Source: CAD feature listing. Evaluate the final solid. Frame: model axes, mm. A direction names the side the tool comes from. Round coordinates to 2 decimals unless told otherwise and drop trailing zeros. Write each loop counter-clockwise with the first axis right and the second up, starting at its lowest first coordinate (ties: lowest second). Pieces come first, ordered by that corner, then holes. Notation, with made-up numbers: M 8,55 L 33,55 A10 ccw 33,64 Z; hole C 48,54.25 d3. An arc over 180 degrees is marked long. Put each result on its own line as item: value. Start each with the question number.
```python
from build123d import *

# Parameters (mm, degrees)
SKETCH1_W           = 132
SKETCH1_H           = 87
SKETCH1_W_2         = 100
SKETCH1_H_2         = 55
BOSS_EXTRUDE1_DEPTH = 256
CUT_EXTRUDE1_REACH  = 89
SKETCH4_W           = 80
SKETCH4_H           = 70
CUT_EXTRUDE2_REACH  = 89
SKETCH5_W           = 70
SKETCH5_H           = 70
SKETCH6_W           = 100
SKETCH6_H           = 55
BOSS_EXTRUDE2_DEPTH = 16
SKETCH7_W           = 106
SKETCH7_H           = 17.5
CUT_EXTRUDE3_DEPTH  = 133
SKETCH9_W           = 106
SKETCH9_H           = 7.5
BOSS_EXTRUDE4_DEPTH = 16
CUT_EXTRUDE4_REACH  = 134
SKETCH10_R          = 12.5


with BuildPart() as part:
    # Sketch1 → Boss-Extrude1 (new body)
    with BuildSketch(Plane.XY):
        with Locations((-66, 43.5)):
            Rectangle(SKETCH1_W, SKETCH1_H)
        with Locations((-66, 43.5)):
            Rectangle(SKETCH1_W_2, SKETCH1_H_2, mode=Mode.SUBTRACT)
    extrude(amount=BOSS_EXTRUDE1_DEPTH)

    # Sketch4 → Cut-Extrude1 (cut, up to next)
    with BuildSketch(Plane(origin=(0, 87, 0), x_dir=(1, 0, 0), z_dir=(0, 1, 0)), mode=Mode.PRIVATE) as cut_extrude1_sk1:
        with Locations((-66, -201)):
            Rectangle(SKETCH4_W, SKETCH4_H)
    cut_extrude1_tool1 = extrude(cut_extrude1_sk1.sketch, amount=-CUT_EXTRUDE1_REACH, mode=Mode.PRIVATE) & part.part
    add(cut_extrude1_tool1.solids().sort_by_distance((-66, 87, 201))[0], mode=Mode.SUBTRACT)

    # Sketch5 → Cut-Extrude2 (cut, up to next)
    with BuildSketch(Plane(origin=(0, 87, 0), x_dir=(1, 0, 0), z_dir=(0, 1, 0)), mode=Mode.PRIVATE) as cut_extrude2_sk1:
        with Locations((-66, -51)):
            Rectangle(SKETCH5_W, SKETCH5_H)
    cut_extrude2_tool1 = extrude(cut_extrude2_sk1.sketch, amount=-CUT_EXTRUDE2_REACH, mode=Mode.PRIVATE) & part.part
    add(cut_extrude2_tool1.solids().sort_by_distance((-66, 87, 51))[0], mode=Mode.SUBTRACT)

    # Sketch6 → Boss-Extrude2 (add)
    with BuildSketch(Plane(origin=(0, 0, 0), x_dir=(-1, 0, 0), z_dir=(0, 0, -1))):
        with Locations((66, 43.5)):
            Rectangle(SKETCH6_W, SKETCH6_H)
    extrude(amount=-BOSS_EXTRUDE2_DEPTH)

    # Sketch7 → Cut-Extrude3 (cut, through all)
    with BuildSketch(Plane(origin=(0, 0, 0), x_dir=(0, 0, -1), z_dir=(1, 0, 0))):
        with Locations((-53, 8.75)):
            Rectangle(SKETCH7_W, SKETCH7_H)
    extrude(amount=-CUT_EXTRUDE3_DEPTH, mode=Mode.SUBTRACT)

    # Sketch9 → Boss-Extrude4 (add)
    with BuildSketch(Plane.ZY.offset(132)):
        with Locations((53, 13.75)):
            Rectangle(SKETCH9_W, SKETCH9_H)
    extrude(amount=-BOSS_EXTRUDE4_DEPTH)

    # Sketch10 → Cut-Extrude4 (cut, up to next)
    with BuildSketch(Plane.ZY.offset(132), mode=Mode.PRIVATE) as cut_extrude4_sk1:
        with Locations((201, 57.5)):
            Circle(SKETCH10_R)
    cut_extrude4_tool1 = extrude(cut_extrude4_sk1.sketch, amount=-CUT_EXTRUDE4_REACH, mode=Mode.PRIVATE) & part.part
    add(cut_extrude4_tool1.solids().sort_by_distance((-132, 57.5, 201))[0], mode=Mode.SUBTRACT)


solid = part.part
```
(1) Section query B-B (x = -18.5). Return loops of the section in (y, z), and give its area (3 significant figures).
(2) Pull-direction query (X, two-part tool) for faces 1 (the flat face through (-67, 87, 126)), 2 (the flat face through (-67, 53, 16)), 3 (the flat face through (-132, 44, 126)); classes: +X half, -X half, draft (parallel to the pull), parting line (faces both ways), or undercut.
(3) Ray query, line 1 along X through (y, z) = (58, 136); line 2 along Y through (x, z) = (-127, 201); line 3 along Y through (x, z) = (-71.5, 130.5). Return the intervals inside material, ascending.
(4) Section query D-D (x = -44). Return loops of the section in (y, z).
(5) Access query for faces 4 (the flat face through (-67, 16, 180)), 5 (the flat face through (-124, 10, 52)), 6 (the flat face through (-67, 71, 161)). Directions: +Z, -Z, +X, -X, +Y, -Y. A direction counts if a zero-diameter tool reaches every point of the face in a straight line with its end or side. Return the directions, or none.
(6) Contact query for flat-ended pins moving along their axis: P1, Ø13, axis at x = -61, y = 83, coming from the -Z side; P2, Ø19, axis at x = -67, y = 5.5, coming from the -Z side; P3, Ø2, axis at x = -100.5, y = 34.5, coming from the +Z side; P4, Ø5, axis at x = -58.5, z = 200, coming from the +Y side. Output: stop coordinate, or through.
(7) Section query C-C (y = 57.5). Return loops of the section in (x, z), and give its area (3 significant figures).
(8) Section query A-A (z = 201). Return loops of the section in (x, y), and give its area (3 significant figures).
Entries:
1. outline: M 0,106 L 16,106 L 16,256 L 0,256 Z; M 17.5,0 L 87,0 L 87,256 L 71,256 L 71,16 L 17.5,16 Z
1. area: 7,350 mm2
2. face 1: draft
2. face 2: undercut
2. face 3: -X half
3. line 1: -132 to -116, -16 to 0
3. line 2: 0 to 45, 70 to 87
3. line 3: 0 to 16, 71 to 87
4. outline: M 0,106 L 16,106 L 16,256 L 0,256 Z; M 17.5,0 L 87,0 L 87,16 L 17.5,16 Z; M 71,86 L 87,86 L 87,166 L 71,166 Z; M 71,236 L 87,236 L 87,256 L 71,256 Z
5. face 4: +Z, -Z
5. face 5: -Z, +X, -X, -Y
5. face 6: +Z
6. P1: z = 0
6. P2: z = 106
6. P3: z = 16
6. P4: y = 16
7. outline: M -132,0 L 0,0 L 0,256 L -16,256 L -16,16 L -116,16 L -116,188.5 L -132,188.5 Z; M -132,213.5 L -116,213.5 L -116,256 L -132,256 Z
7. area: 9,390 mm2
8. outline: M -132,0 L 0,0 L 0,87 L -26,87 L -26,71 L -16,71 L -16,16 L -116,16 L -116,45 L -132,45 Z; M -132,70 L -116,70 L -116,71 L -106,71 L -106,87 L -132,87 Z
8. area: 4,300 mm2
